Drawing for the job (mm, zero at the part's lowest x, y, z). A direction names the side the tool comes from. Round coordinates to 2 decimals unless told otherwise and drop trailing zeros. Write each loop counter-clockwise with the first axis right and the second up, starting at its lowest first coordinate (ties: lowest second). Pieces come first, ordered by that corner, then holes. Notation, with made-up numbers: (46, 85) - (93, 85) arc R10 ccw to (93, 101) - close; hole circle Ø2 at (46, 7.5). An arc over 180 degrees is marked (long way). One line per question, with ' | ' between items.
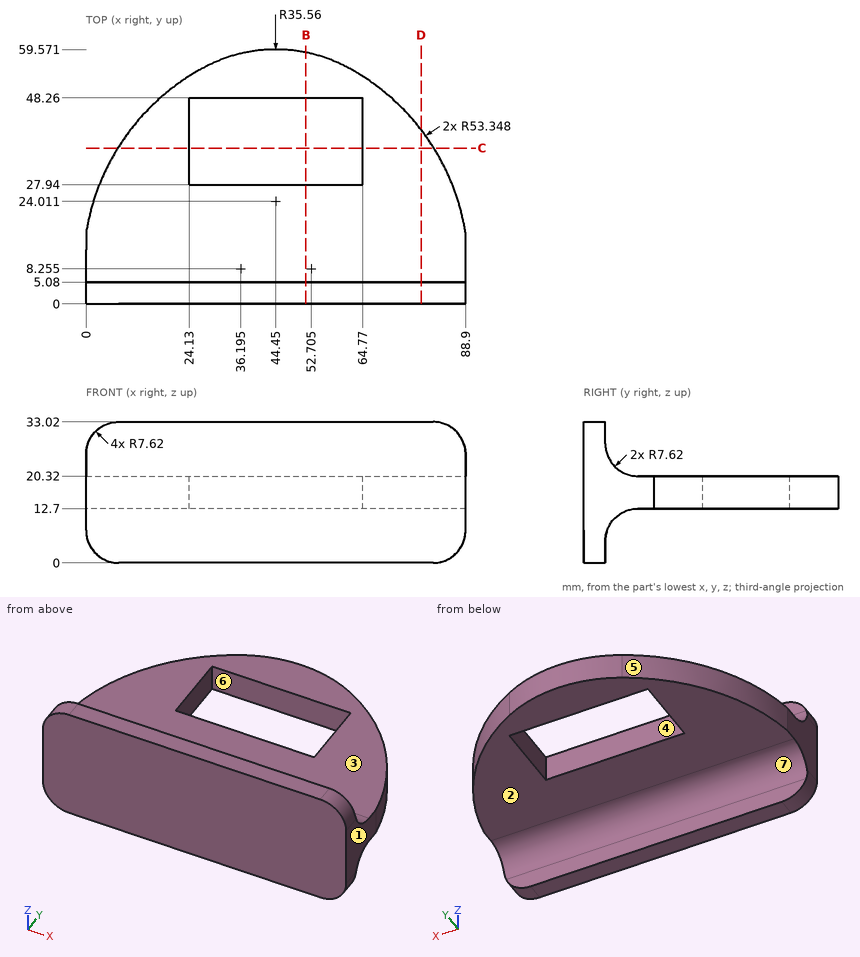
Q1. Drill centre lines: L1, parallel to Z at x = 60.5, y = 13.5; L2, parallel to Y at x = 4, z = 5.5; L3, parallel to X at y = 48, z = 16. Where is each one in solid material? Low to high. Write a range as from..to.
Found:
L1: 12.7..20.32 | L2: 0..5.09 | L3: 17.12..24.13, 64.77..71.78
Q2. Pull direction X, two halves, no side cores. Call the marked faces 4, 5, 6 and 7: +X half, -X half, draft (parallel to the pull), parting line (faces both ways), or undercut.
Found:
face 4: undercut | face 5: -X half | face 6: undercut | face 7: draft
Q3. Drop flat-ended pins along their axis: pin 1 (1.5 mm diameter, centred on x = 61.5, z = 29.5, fed in from +Y); pin 2 (4 mm diameter, centred on x = 68.5, y = 48.5, fed in from -Z); pin 3 (1 mm diameter, centred on y = 48.5, z = 20, fed in from -X). Give the stop position or say it passes through.
Found:
pin 1: y = 5.08 | pin 2: z = 12.7 | pin 3: x = 17.12
Q4. Saw through at B-B, the plane x = 51.5. List the corners of the cut face in (y, z) (1 decimal).
Found:
outline: (0, 0) - (5.1, 0) - (5.1, 5.1) arc R7.6 cw to (12.7, 12.7) - (27.9, 12.7) - (27.9, 20.3) - (12.7, 20.3) arc R7.6 cw to (5.1, 27.9) - (5.1, 33) - (0, 33) - close; (48.3, 12.7) - (58.9, 12.7) - (58.9, 20.3) - (48.3, 20.3) - close
Q5. Saw through at C-C, the plane y = 36.5. List the corners of the cut face in (x, z).
Found:
outline: (7.45, 12.7) - (24.13, 12.7) - (24.13, 20.32) - (7.45, 20.32) - close; (64.77, 12.7) - (81.45, 12.7) - (81.45, 20.32) - (64.77, 20.32) - close
Q6. Saw through at D-D, the plane x = 78.5. List the corners of the cut face in (y, z) (1 decimal).
Found:
outline: (0, 0) - (5.1, 0) - (5.1, 5.1) arc R7.6 cw to (12.7, 12.7) - (40.8, 12.7) - (40.8, 20.3) - (12.7, 20.3) arc R7.6 cw to (5.1, 27.9) - (5.1, 33) - (0, 33) - close
Q7. Which spindle directions (+Z, -Z, +X, -X, +Y, -Y) get a long thin tool onto all of the face, cutting with end or side? Do the marked faces 1, 2 and 3. Say none if no direction does.
Found:
face 1: +Z, -Z, +X, +Y, -Y | face 2: -Z, +X, -X, +Y | face 3: +Z, +X, -X, +Y
